Geometry check sheet. Reference: drawing and pictorial views, mm from the part's lowest x, y, z. A direction names the side the tool comes from. Give positions to 0.01 mm unless a question says otherwise; leave off trailing zeros. Write each loop counter-clockwise with the first axis right and the second up, starting at its lowest first coordinate (ties: lowest second). Pieces come first, ordered by that corner, then holes. Notation, with made-up numbers: (65, -9) -> (110, -9) arc R18 ccw to (110, 6) -> close; hole circle Ø6 at (-7, 61). An arc over 180 degrees is marked (long way). Use a Markdown table: item, result. Add a question column.
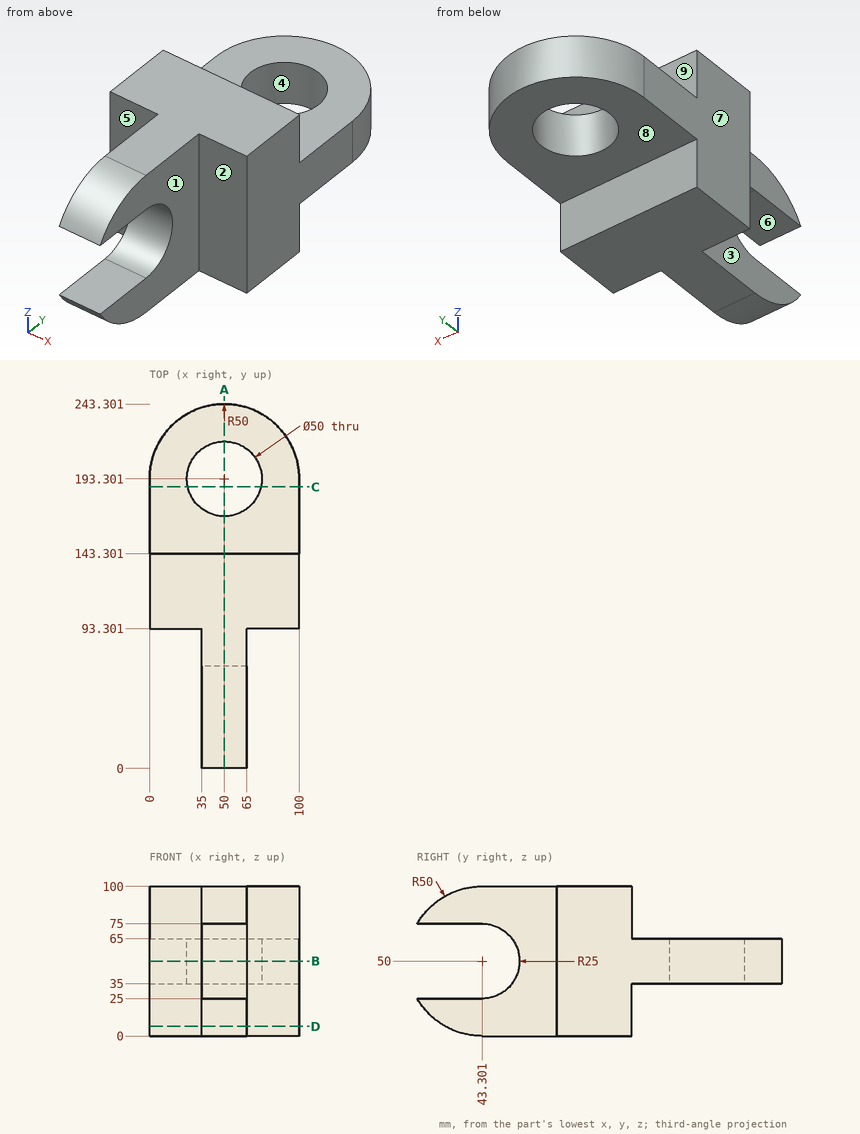
1) Sectioned sample at D-D, the plane z = 6.5. Enter the section's corners in (x, y), and give its area (3 significant figures).
2) Sectioned sample at B-B, the plane z = 50. Enter the section's corners in (x, y).
3) Sectioned sample at A-A, the plane x = 50. Enter the section's corners in (y, z).
4) Draft check along X on the marked faces 1, 2, 3 and 4. Enter one of: +X half, -X half, draft (parallel to the pull), parting line (faces both ways), or undercut.
5) Gauge pin test, flat ends, axial feed: P1, Ø1, axis at x = 74.5, z = 20.5, coming from the +Y side; P2, Ø8, axis at x = 14.5, y = 160, coming from the +Z side; P3, Ø4, axis at x = 32.5, z = 44.5, coming from the -Y side. Record the tip position at first contact, or that the pin passes through.
6) Tool access check on the marked faces 5, 6, 7, 8 and 9. Record the directions out of +Z, -Z, +X, -X, +Y, -Y that give a thin tool (end or side, any length) a straight path to the whole face; none if there is none.
7) Material ranges on probe 1 along Y at (x, z) = (89, 92.5); probe 2 along Y at (x, z) = (50, 51); probe 3 along X at (y, z) = (176.5, 47), recorded low to high. Write a range as [from, to].
8) Sectioned sample at C-C, the plane y = 188. Enter the section's corners in (x, z).
Check values:
| question | item | result |
|---|---|---|
| 1 | outline | (0, 93.3) -> (35, 93.3) -> (35, 18.65) -> (65, 18.65) -> (65, 93.3) -> (100, 93.3) -> (100, 143.3) -> (0, 143.3) -> close |
| 1 | area | 7,240 mm² |
| 2 | outline | (0, 93.3) -> (35, 93.3) -> (35, 68.3) -> (65, 68.3) -> (65, 93.3) -> (100, 93.3) -> (100, 193.3) arc R50 ccw to (0, 193.3) -> close; hole circle Ø50 at (50, 193.3) |
| 3 | outline | (0, 25) arc R50 ccw to (43.3, 0) -> (143.3, 0) -> (143.3, 35) -> (168.3, 35) -> (168.3, 65) -> (143.3, 65) -> (143.3, 100) -> (43.3, 100) arc R50 ccw to (0, 75) -> (43.3, 75) arc R25 cw to (43.3, 25) -> close; (218.3, 35) -> (243.3, 35) -> (243.3, 65) -> (218.3, 65) -> close |
| 4 | face 1 | +X half |
| 4 | face 2 | draft |
| 4 | face 3 | -X half |
| 4 | face 4 | undercut |
| 5 | P1 | y = 143.3 |
| 5 | P2 | z = 65 |
| 5 | P3 | y = 93.3 |
| 6 | face 5 | +Z, -Z, -X, -Y |
| 6 | face 6 | +X, -X, -Y |
| 6 | face 7 | +Z, -Z, -X, +Y, -Y |
| 6 | face 8 | -Z, +X, -X, +Y |
| 6 | face 9 | +Z, +X, -X, +Y |
| 7 | probe 1 | [93.3, 143.3] |
| 7 | probe 2 | [68.28, 168.3], [218.3, 243.3] |
| 7 | probe 3 | [0, 31.49], [68.51, 100] |
| 8 | outline | (0, 35) -> (25.57, 35) -> (25.57, 65) -> (0, 65) -> close; (74.43, 35) -> (100, 35) -> (100, 65) -> (74.43, 65) -> close |
